from build123d import *

# Parameters (mm, degrees)
SKETCH1_R           = 1.5
BOSS_EXTRUDE1_DEPTH = 9.65
CUT_EXTRUDE1_START  = -1
SKETCH2_R           = 1.5
CUT_EXTRUDE1_DEPTH  = 1
SKETCH4_W           = 12.876
SKETCH4_H           = 8
CUT_EXTRUDE2_DEPTH  = 3


with BuildPart() as part:
    # Sketch1 → Boss-Extrude1 (new body)
    with BuildSketch(Plane(origin=(0, 0, 0), x_dir=(1, 0, 0), z_dir=(0, 1, 0))):
        with BuildLine():
            Line((2.75, 0), (35.35, 0))
            ThreePointArc((35.35, 0), (37.294543648, -0.805456352), (38.1, -2.75))
            Line((38.1, -2.75), (38.1, -21.126))
            ThreePointArc((38.1, -21.126), (37.294543648, -23.070543648), (35.35, -23.876))
            Line((35.35, -23.876), (2.75, -23.876))
            ThreePointArc((2.75, -23.876), (0.805456352, -23.070543648), (0, -21.126))
            Line((0, -21.126), (0, -2.75))
            ThreePointArc((0, -2.75), (0.805456352, -0.805456352), (2.75, 0))
        make_face()
        with Locations(Location((2.75, -2.75, 0), (0, 0, 270))):
            Circle(SKETCH1_R, mode=Mode.SUBTRACT)
        with Locations(Location((2.75, -21.126, 0), (0, 0, 270))):
            Circle(SKETCH1_R, mode=Mode.SUBTRACT)
        with Locations(Location((35.35, -11.938, 0), (0, 0, 270))):
            Circle(SKETCH1_R, mode=Mode.SUBTRACT)
    extrude(amount=BOSS_EXTRUDE1_DEPTH)

    # Sketch2 → Cut-Extrude1 (cut)
    # profile 1 of 20: a face of its own
    with BuildSketch(Plane(origin=(0, 9.65, 0), x_dir=(1, 0, 0), z_dir=(0, 1, 0)).offset(CUT_EXTRUDE1_START)):
        with BuildLine():
            Line((2.75, -18.376), (0, -18.376))
            Line((0, -18.376), (0, -21.126))
            ThreePointArc((0, -21.126), (0.805456352, -19.181456352), (2.75, -18.376))
        make_face()
    # profile 2 of 20: a face of its own
    with BuildSketch(Plane(origin=(0, 9.65, 0), x_dir=(1, 0, 0), z_dir=(0, 1, 0)).offset(CUT_EXTRUDE1_START)):
        with BuildLine():
            ThreePointArc((2.75, -23.876), (0.805456352, -23.070543648), (0, -21.126))
            Line((0, -21.126), (0, -23.876))
            Line((0, -23.876), (2.75, -23.876))
        make_face()
    # profile 3 of 20: a face of its own
    with BuildSketch(Plane(origin=(0, 9.65, 0), x_dir=(1, 0, 0), z_dir=(0, 1, 0)).offset(CUT_EXTRUDE1_START)):
        with BuildLine():
            ThreePointArc((5.5, -21.126), (4.694543648, -19.181456352), (2.75, -18.376))
            ThreePointArc((2.75, -18.376), (0.805456352, -19.181456352), (0, -21.126))
            ThreePointArc((0, -21.126), (0.805456352, -23.070543648), (2.75, -23.876))
            ThreePointArc((2.75, -23.876), (4.694543648, -23.070543648), (5.5, -21.126))
        make_face()
        with Locations(Location((2.75, -21.126, 0), (0, 0, 270))):
            Circle(SKETCH2_R, mode=Mode.SUBTRACT)
    # profile 4 of 20: a face of its own
    with BuildSketch(Plane(origin=(0, 9.65, 0), x_dir=(1, 0, 0), z_dir=(0, 1, 0)).offset(CUT_EXTRUDE1_START)):
        with Locations(Location((2.75, -21.126, 0), (0, 0, 270))):
            Circle(SKETCH2_R)
    # profile 5 of 20: a face of its own
    with BuildSketch(Plane(origin=(0, 9.65, 0), x_dir=(1, 0, 0), z_dir=(0, 1, 0)).offset(CUT_EXTRUDE1_START)):
        with BuildLine():
            Line((5.5, -23.876), (5.5, -21.126))
            ThreePointArc((5.5, -21.126), (4.694543648, -23.070543648), (2.75, -23.876))
            Line((2.75, -23.876), (5.5, -23.876))
        make_face()
    # profile 6 of 20: a face of its own
    with BuildSketch(Plane(origin=(0, 9.65, 0), x_dir=(1, 0, 0), z_dir=(0, 1, 0)).offset(CUT_EXTRUDE1_START)):
        with BuildLine():
            ThreePointArc((0, -2.75), (0.805456352, -4.694543648), (2.75, -5.5))
            ThreePointArc((2.75, -5.5), (4.694543648, -4.694543648), (5.5, -2.75))
            ThreePointArc((5.5, -2.75), (4.694543648, -0.805456352), (2.75, 0))
            ThreePointArc((2.75, 0), (0.805456352, -0.805456352), (0, -2.75))
        make_face()
        with Locations(Location((2.75, -2.75, 0), (0, 0, 270))):
            Circle(SKETCH2_R, mode=Mode.SUBTRACT)
    # profile 7 of 20: a face of its own
    with BuildSketch(Plane(origin=(0, 9.65, 0), x_dir=(1, 0, 0), z_dir=(0, 1, 0)).offset(CUT_EXTRUDE1_START)):
        with Locations(Location((2.75, -2.75, 0), (0, 0, 270))):
            Circle(SKETCH2_R)
    # profile 8 of 20: a face of its own
    with BuildSketch(Plane(origin=(0, 9.65, 0), x_dir=(1, 0, 0), z_dir=(0, 1, 0)).offset(CUT_EXTRUDE1_START)):
        with BuildLine():
            Line((0, -5.5), (2.75, -5.5))
            ThreePointArc((2.75, -5.5), (0.805456352, -4.694543648), (0, -2.75))
            Line((0, -2.75), (0, -5.5))
        make_face()
    # profile 9 of 20: a face of its own
    with BuildSketch(Plane(origin=(0, 9.65, 0), x_dir=(1, 0, 0), z_dir=(0, 1, 0)).offset(CUT_EXTRUDE1_START)):
        with BuildLine():
            Line((0, 0), (0, -2.75))
            ThreePointArc((0, -2.75), (0.805456352, -0.805456352), (2.75, 0))
            Line((2.75, 0), (0, 0))
        make_face()
    # profile 10 of 20: a face of its own
    with BuildSketch(Plane(origin=(0, 9.65, 0), x_dir=(1, 0, 0), z_dir=(0, 1, 0)).offset(CUT_EXTRUDE1_START)):
        with BuildLine():
            ThreePointArc((2.75, 0), (4.694543648, -0.805456352), (5.5, -2.75))
            Line((5.5, -2.75), (5.5, 0))
            Line((5.5, 0), (2.75, 0))
        make_face()
    # profile 11 of 20: a face of its own
    with BuildSketch(Plane(origin=(0, 9.65, 0), x_dir=(1, 0, 0), z_dir=(0, 1, 0)).offset(CUT_EXTRUDE1_START)):
        with BuildLine():
            ThreePointArc((38.1, -11.938), (37.294543648, -9.993456352), (35.35, -9.188))
            Line((35.35, -9.188), (35.35, -10.438))
            ThreePointArc((35.35, -10.438), (36.410660172, -10.877339828), (36.85, -11.938))
            ThreePointArc((36.85, -11.938), (36.410660172, -12.998660172), (35.35, -13.438))
            Line((35.35, -13.438), (35.35, -14.688))
            ThreePointArc((35.35, -14.688), (37.294543648, -13.882543648), (38.1, -11.938))
        make_face()
    # profile 12 of 20: a face of its own
    with BuildSketch(Plane(origin=(0, 9.65, 0), x_dir=(1, 0, 0), z_dir=(0, 1, 0)).offset(CUT_EXTRUDE1_START)):
        with BuildLine():
            Line((35.35, -10.438), (35.35, -9.188))
            ThreePointArc((35.35, -9.188), (32.6, -11.938), (35.35, -14.688))
            Line((35.35, -14.688), (35.35, -13.438))
            ThreePointArc((35.35, -13.438), (33.85, -11.938), (35.35, -10.438))
        make_face()
    # profile 13 of 20: a face of its own
    with BuildSketch(Plane(origin=(0, 9.65, 0), x_dir=(1, 0, 0), z_dir=(0, 1, 0)).offset(CUT_EXTRUDE1_START)):
        with BuildLine():
            ThreePointArc((36.85, -11.938), (36.410660172, -10.877339828), (35.35, -10.438))
            Line((35.35, -10.438), (35.35, -13.438))
            ThreePointArc((35.35, -13.438), (36.410660172, -12.998660172), (36.85, -11.938))
        make_face()
    # profile 14 of 20: a face of its own
    with BuildSketch(Plane(origin=(0, 9.65, 0), x_dir=(1, 0, 0), z_dir=(0, 1, 0)).offset(CUT_EXTRUDE1_START)):
        with BuildLine():
            Line((35.35, -13.438), (35.35, -10.438))
            ThreePointArc((35.35, -10.438), (33.85, -11.938), (35.35, -13.438))
        make_face()
    # profile 15 of 20: a face of its own
    with BuildSketch(Plane(origin=(0, 9.65, 0), x_dir=(1, 0, 0), z_dir=(0, 1, 0)).offset(CUT_EXTRUDE1_START)):
        with BuildLine():
            ThreePointArc((36.85, -11.938), (36.410660172, -10.877339828), (35.35, -10.438))
            Line((35.35, -10.438), (35.35, -13.438))
            ThreePointArc((35.35, -13.438), (36.410660172, -12.998660172), (36.85, -11.938))
        make_face()
    # profile 16 of 20: a face of its own
    with BuildSketch(Plane(origin=(0, 9.65, 0), x_dir=(1, 0, 0), z_dir=(0, 1, 0)).offset(CUT_EXTRUDE1_START)):
        with BuildLine():
            Line((35.35, -13.438), (35.35, -10.438))
            ThreePointArc((35.35, -10.438), (33.85, -11.938), (35.35, -13.438))
        make_face()
    # profile 17 of 20: a face of its own
    with BuildSketch(Plane(origin=(0, 9.65, 0), x_dir=(1, 0, 0), z_dir=(0, 1, 0)).offset(CUT_EXTRUDE1_START)):
        with BuildLine():
            ThreePointArc((38.1, -11.938), (37.294543648, -9.993456352), (35.35, -9.188))
            Line((35.35, -9.188), (35.35, -10.438))
            ThreePointArc((35.35, -10.438), (36.410660172, -10.877339828), (36.85, -11.938))
            ThreePointArc((36.85, -11.938), (36.410660172, -12.998660172), (35.35, -13.438))
            Line((35.35, -13.438), (35.35, -14.688))
            ThreePointArc((35.35, -14.688), (37.294543648, -13.882543648), (38.1, -11.938))
        make_face()
    # profile 18 of 20: a face of its own
    with BuildSketch(Plane(origin=(0, 9.65, 0), x_dir=(1, 0, 0), z_dir=(0, 1, 0)).offset(CUT_EXTRUDE1_START)):
        with BuildLine():
            Line((35.35, -10.438), (35.35, -9.188))
            ThreePointArc((35.35, -9.188), (32.6, -11.938), (35.35, -14.688))
            Line((35.35, -14.688), (35.35, -13.438))
            ThreePointArc((35.35, -13.438), (33.85, -11.938), (35.35, -10.438))
        make_face()
    # profile 19 of 20: a face of its own
    with BuildSketch(Plane(origin=(0, 9.65, 0), x_dir=(1, 0, 0), z_dir=(0, 1, 0)).offset(CUT_EXTRUDE1_START)):
        with BuildLine():
            Line((38.1, -14.688), (38.1, -11.938))
            ThreePointArc((38.1, -11.938), (37.294543648, -13.882543648), (35.35, -14.688))
            Line((35.35, -14.688), (38.1, -14.688))
        make_face()
    # profile 20 of 20: a face of its own
    with BuildSketch(Plane(origin=(0, 9.65, 0), x_dir=(1, 0, 0), z_dir=(0, 1, 0)).offset(CUT_EXTRUDE1_START)):
        with BuildLine():
            Line((38.1, -9.188), (35.35, -9.188))
            ThreePointArc((35.35, -9.188), (37.294543648, -9.993456352), (38.1, -11.938))
            Line((38.1, -11.938), (38.1, -9.188))
        make_face()
    extrude(amount=CUT_EXTRUDE1_DEPTH, mode=Mode.SUBTRACT)

    # Sketch4 → Cut-Extrude2 (cut)
    with BuildSketch(Plane.ZY):
        with Locations((11.938, 4)):
            Rectangle(SKETCH4_W, SKETCH4_H)
    extrude(amount=-CUT_EXTRUDE2_DEPTH, mode=Mode.SUBTRACT)


solid = part.part
Geometry: final body of the model. Coordinates: model frame, mm. A direction names the side the tool comes from. Coordinates: 2 decimals unless noted, no trailing zeros. Order: outer loops, then holes, each group sorted by start corner. A loop starts at its lowest first (then second) coordinate and runs counter-clockwise, first axis right, second up.
1) First-contact query: P1, Ø0.8, axis at x = 2, y = 9, coming from the -Z side; P2, Ø3, axis at y = 3, z = 10, coming from the -X side; P3, Ø0.8, axis at y = 9.5, z = 22.5, coming from the -X side; P4, Ø2, axis at x = 11, z = 15.5, coming from the -Y side. Flat tips, straight axial feed; report the tip coordinate or a pass-through.
Result sheet:
P1: stops at z = 0.06
P2: stops at x = 3
P3: stops at x = 5.5
P4: stops at y = 0
2) Set-up query: faces 4 (the cylindrical face through (32.6, 9.1, 11.9)), 5 (the flat face through (5.5, 9, 23)), 6 (the flat face through (1, 4, 5.5)). Return all of +Z, -Z, +X, -X, +Y, -Y with unobstructed straight access to the full face (end or side cutting, diameter ignored); none if empty.
Result sheet:
face 4: +X, +Y
face 5: +Z, -X, +Y
face 6: -X, -Y
3) Draft query along X for faces 1 (the cylindrical face through (35.8, 4.26, 13.37)), 2 (the flat face through (3, 4, 12)), 3 (the flat face through (1, 4, 18.376)). Return one class per face: released by +X, released by -X, zero draft, split by the parting line, or undercut.
Result sheet:
face 1: undercut
face 2: released by -X
face 3: zero draft
4) Section B-B (z = 20.25). Return loops of the section in (x, y), then the cut area to 3 significant figures.
Result sheet:
outline: (0, 0) - (1.53, 0) - (1.53, 8.65) - (0, 8.65) - close; (3.97, 0) - (38.1, 0) - (38.1, 9.65) - (5.36, 9.65) - (5.36, 8.65) - (3.97, 8.65) - close
area: 341 mm2
5) Section A-A (y = 2.25). Return loops of the section in (x, z), then the cut area to 3 significant figures.
Result sheet:
outline: (0, 2.75) arc R2.75 ccw to (2.75, 0) - (35.35, 0) arc R2.75 ccw to (38.1, 2.75) - (38.1, 21.13) arc R2.75 ccw to (35.35, 23.88) - (2.75, 23.88) arc R2.75 ccw to (0, 21.13) - (0, 18.38) - (3, 18.38) - (3, 5.5) - (0, 5.5) - close; hole circle Ø3 at (2.75, 2.75); hole circle Ø3 at (2.75, 21.13); hole circle Ø3 at (35.35, 11.94)
area: 843 mm2
6) Ray query, probe 1 along X at (y, z) = (3, 2.75); probe 2 along Z at (x, y) = (4, 4); probe 3 along X at (y, z) = (4.25, 22). Return the intervals inside material, ascending.
Result sheet:
probe 1: x = 0 to 1.25, 4.25 to 38.1
probe 2: z = 0 to 1.92, 3.58 to 20.3, 21.96 to 23.88
probe 3: x = 0.14 to 1.53, 3.97 to 37.96
